Check sheet for the modelled part. Datum: model origin and axes. Units: mm. A direction names the side the tool comes from. Coordinates: 2 decimals unless noted, no trailing zeros. Write each loop counter-clockwise with the first axis right and the second up, starting at its lowest first coordinate (ties: lowest second). Pieces come first, ordered by that corner, then holes. Notation, with made-up numbers: (43.5, 6) -> (67.5, 6) arc R28 ccw to (67.5, 40) -> close; hole circle Ø4 at (63.25, 25). An arc over 180 degrees is marked (long way). One line per item, written item: value. Start each with the question number.
1) Sectioned sample at C-C on y = -4.75. Give the number of separate pieces and of enclosed holes in the cut face, plus the area to 3 significant figures.
2) Gauge pin test, flat ends, axial feed: P1, Ø1.5, axis at x = -12, y = -15, coming from the -Z side; P2, Ø4, axis at x = 34.5, z = -45.5, coming from the -Y side; P3, Ø8, axis at x = 9, y = -6.5, coming from the +Z side. Record the tip position at first contact, or that the pin passes through.
3) Scan lines: line 1 along Z through (x, y) = (0, -0.3); line 2 along X through (y, z) = (-17.75, -22.5); line 3 along Z through (x, y) = (-41, -12). Record each from-to range of solid material in increasing order. Write a range as [from, to].
4) Sectioned sample at D-D on x = -44. Enter the section's corners in (y, z).
5) Sectioned sample at B-B on z = 0. Enter the section's corners in (x, y).
6) Draft check along Z on faces 1 (the cylindrical face through (-35.48, -12.83, 51.01)), 2 (the flat face through (30, -25, 40)), 3 (the flat face through (43.919, -12.832, 3.362)). Enter one of: +Z half, -Z half, draft (parallel to the pull), parting line (faces both ways), or undercut.
7) Sectioned sample at A-A on x = 0. Enter the section's corners in (y, z), plus the area to 3 significant figures.
8) Set-up check for faces 4 (the flat face through (-34.05, -12.83, -27.95)), 5 (the flat face through (10, -13, 43)), 6 (the cylindrical face through (27.912, -13.168, -19.875)), 7 (the flat face through (-23, -25, -30)): record each of +Z, -Z, +X, -X, +Y, -Y from which the full face is reachable in a straight line by a thin tool's end or side.
```python
from build123d import *

# Parameters (mm, degrees)
F0_R     = 68.635064
F0_R_2   = 2.1
F0_R_3   = 28.5
F1_DEPTH = 1
F2_DEPTH = 25
F3_R     = 10


with BuildPart() as f1:
    # F0 (on Front) → F1 (new body)
    with BuildSketch(Plane.XZ):
        Circle(F0_R)
        with Locations((-22.828554, -29.75075)):
            Circle(F0_R_2, mode=Mode.SUBTRACT)
        with Locations((21.509116, -30.718202)):
            Circle(F0_R_2, mode=Mode.SUBTRACT)
        with BuildLine():
            ThreePointArc((-10, 30.923292), (0, 32.5), (10, 30.923292))
            Line((10, 30.923292), (10, 61.325086))
            ThreePointArc((10, 61.325086), (36.741063, 50.108487), (55.479716, 27.977979))
            Line((55.479716, 27.977979), (26.48501, 18.835983))
            ThreePointArc((26.48501, 18.835983), (30.959755, 9.886536), (32.5, 0))
            ThreePointArc((32.5, 0), (32.499781, -0.119179), (32.499126, -0.238356))
            Line((32.499126, -0.238356), (61.493832, 8.90364))
            ThreePointArc((61.493832, 8.90364), (58.837564, -19.972662), (43.366145, -44.498805))
            Line((43.366145, -44.498805), (25.928392, -19.595114))
            ThreePointArc((25.928392, -19.595114), (18.641234, -26.622441), (9.545351, -31.066642))
            Line((9.545351, -31.066642), (26.983104, -55.970334))
            ThreePointArc((26.983104, -55.970334), (-1.355469, -62.120278), (-29.398814, -54.740076))
            Line((-29.398814, -54.740076), (-10.891374, -30.620711))
            ThreePointArc((-10.891374, -30.620711), (-19.784746, -25.783984), (-26.758441, -18.445483))
            Line((-26.758441, -18.445483), (-45.265881, -42.564848))
            ThreePointArc((-45.265881, -42.564848), (-59.652759, -17.387194), (-61.046932, 11.577489))
            Line((-61.046932, 11.577489), (-32.478591, 1.179463))
            ThreePointArc((-32.478591, 1.179463), (-30.54001, 11.115655), (-25.638188, 19.973315))
            Line((-25.638188, 19.973315), (-54.20653, 30.371341))
            ThreePointArc((-54.20653, 30.371341), (-35.639209, 50.898065), (-10, 61.325086))
            Line((-10, 61.325086), (-10, 30.923292))
        make_face(mode=Mode.SUBTRACT)
        with Locations((-35.238473, 12.825755)):
            Circle(F0_R_2, mode=Mode.SUBTRACT)
        with Locations((35.764386, 11.276467)):
            Circle(F0_R_2, mode=Mode.SUBTRACT)
        with Locations((0, 37.5)):
            Circle(F0_R_2, mode=Mode.SUBTRACT)
        with BuildLine():
            Line((10, 61.325086), (10, 30.923292))
            ThreePointArc((10, 30.923292), (19.217564, 26.20945), (26.48501, 18.835983))
            Line((26.48501, 18.835983), (55.479716, 27.977979))
            ThreePointArc((55.479716, 27.977979), (36.741063, 50.108487), (10, 61.325086))
        make_face()
        with BuildLine():
            ThreePointArc((-25.638188, 19.973315), (-18.641234, 26.622441), (-10, 30.923292))
            Line((-10, 30.923292), (-10, 61.325086))
            ThreePointArc((-10, 61.325086), (-35.639209, 50.898065), (-54.20653, 30.371341))
            Line((-54.20653, 30.371341), (-25.638188, 19.973315))
        make_face()
        with Locations((0, 37.5)):
            Circle(F0_R_2)
        with Locations((35.764386, 11.276467)):
            Circle(F0_R_2)
        with BuildLine():
            Line((61.493832, 8.90364), (32.499126, -0.238356))
            ThreePointArc((32.499126, -0.238356), (30.775229, -10.446783), (25.928392, -19.595114))
            Line((25.928392, -19.595114), (43.366145, -44.498805))
            ThreePointArc((43.366145, -44.498805), (58.837564, -19.972662), (61.493832, 8.90364))
        make_face()
        with BuildLine():
            Line((26.983104, -55.970334), (9.545351, -31.066642))
            ThreePointArc((9.545351, -31.066642), (-0.708984, -32.492266), (-10.891374, -30.620711))
            Line((-10.891374, -30.620711), (-29.398814, -54.740076))
            ThreePointArc((-29.398814, -54.740076), (-1.355469, -62.120278), (26.983104, -55.970334))
        make_face()
        with BuildLine():
            ThreePointArc((-26.758441, -18.445483), (-31.20162, -9.094443), (-32.478591, 1.179463))
            Line((-32.478591, 1.179463), (-61.046932, 11.577489))
            ThreePointArc((-61.046932, 11.577489), (-59.652759, -17.387194), (-45.265881, -42.564848))
            Line((-45.265881, -42.564848), (-26.758441, -18.445483))
        make_face()
        with Locations((-35.238473, 12.825755)):
            Circle(F0_R_2)
        with BuildLine():
            ThreePointArc((26.48501, 18.835983), (19.217564, 26.20945), (10, 30.923292))
            ThreePointArc((10, 30.923292), (0, 32.5), (-10, 30.923292))
            ThreePointArc((-10, 30.923292), (-18.641234, 26.622441), (-25.638188, 19.973315))
            ThreePointArc((-25.638188, 19.973315), (-30.54001, 11.115655), (-32.478591, 1.179463))
            ThreePointArc((-32.478591, 1.179463), (-31.20162, -9.094443), (-26.758441, -18.445483))
            ThreePointArc((-26.758441, -18.445483), (-19.784746, -25.783984), (-10.891374, -30.620711))
            ThreePointArc((-10.891374, -30.620711), (-0.708984, -32.492266), (9.545351, -31.066642))
            ThreePointArc((9.545351, -31.066642), (18.641234, -26.622441), (25.928392, -19.595114))
            ThreePointArc((25.928392, -19.595114), (30.775229, -10.446783), (32.499126, -0.238356))
            ThreePointArc((32.499126, -0.238356), (32.499781, -0.119179), (32.5, 0))
            ThreePointArc((32.5, 0), (30.959755, 9.886536), (26.48501, 18.835983))
        make_face()
        Circle(F0_R_3, mode=Mode.SUBTRACT)
        with Locations((21.509116, -30.718202)):
            Circle(F0_R_2)
        with Locations((-22.828554, -29.75075)):
            Circle(F0_R_2)
    extrude(amount=F1_DEPTH)

    # F0 (on Front) → F2 (join)
    with BuildSketch(Plane.XZ):
        with BuildLine():
            Line((10, 61.325086), (10, 30.923292))
            ThreePointArc((10, 30.923292), (19.217564, 26.20945), (26.48501, 18.835983))
            Line((26.48501, 18.835983), (55.479716, 27.977979))
            ThreePointArc((55.479716, 27.977979), (36.741063, 50.108487), (10, 61.325086))
        make_face()
        with BuildLine():
            ThreePointArc((-25.638188, 19.973315), (-18.641234, 26.622441), (-10, 30.923292))
            Line((-10, 30.923292), (-10, 61.325086))
            ThreePointArc((-10, 61.325086), (-35.639209, 50.898065), (-54.20653, 30.371341))
            Line((-54.20653, 30.371341), (-25.638188, 19.973315))
        make_face()
        with BuildLine():
            ThreePointArc((-26.758441, -18.445483), (-31.20162, -9.094443), (-32.478591, 1.179463))
            Line((-32.478591, 1.179463), (-61.046932, 11.577489))
            ThreePointArc((-61.046932, 11.577489), (-59.652759, -17.387194), (-45.265881, -42.564848))
            Line((-45.265881, -42.564848), (-26.758441, -18.445483))
        make_face()
        with BuildLine():
            Line((26.983104, -55.970334), (9.545351, -31.066642))
            ThreePointArc((9.545351, -31.066642), (-0.708984, -32.492266), (-10.891374, -30.620711))
            Line((-10.891374, -30.620711), (-29.398814, -54.740076))
            ThreePointArc((-29.398814, -54.740076), (-1.355469, -62.120278), (26.983104, -55.970334))
        make_face()
        with BuildLine():
            Line((61.493832, 8.90364), (32.499126, -0.238356))
            ThreePointArc((32.499126, -0.238356), (30.775229, -10.446783), (25.928392, -19.595114))
            Line((25.928392, -19.595114), (43.366145, -44.498805))
            ThreePointArc((43.366145, -44.498805), (58.837564, -19.972662), (61.493832, 8.90364))
        make_face()
        with Locations((35.764386, 11.276467)):
            Circle(F0_R_2)
        with Locations((21.509116, -30.718202)):
            Circle(F0_R_2)
        with Locations((-22.828554, -29.75075)):
            Circle(F0_R_2)
        with Locations((-35.238473, 12.825755)):
            Circle(F0_R_2)
        with Locations((0, 37.5)):
            Circle(F0_R_2)
    extrude(amount=F2_DEPTH)

    # F3
    f3_edges = [f1.edges().sort_by_distance(p)[0] for p in [
        (-54.20653, -13, 30.371341),
        (-25.638188, -13, 19.973315),
        (-10, -13, 30.923292),
        (-10, -13, 61.325086),
        (-32.478591, -13, 1.179463),
        (-26.758441, -13, -18.445483),
        (-61.046932, -13, 11.577489),
        (-45.265881, -13, -42.564848),
        (-29.398814, -13, -54.740076),
        (26.983104, -13, -55.970334),
        (9.545351, -13, -31.066642),
        (-10.891374, -13, -30.620711),
        (32.499126, -13, -0.238356),
        (25.928392, -13, -19.595114),
        (43.366145, -13, -44.498805),
        (61.493832, -13, 8.90364),
        (55.479716, -13, 27.977979),
        (10, -13, 61.325086),
        (10, -13, 30.923292),
        (26.48501, -13, 18.835983),
    ]]
    fillet(f3_edges, radius=F3_R)


solid = f1.part
```
Answers:
1. separate pieces: 10
1. enclosed holes: 0
1. area: 5,390 mm2
2. P1: stops at z = -61.11
2. P2: stops at y = -1
2. P3: stops at z = 55.29
3. line 1: z = [-68.64, -28.5], [28.5, 68.64]
3. line 2: x = [-57.92, -29.99], [28.44, 57.92]
3. line 3: z = [-35.11, 4.28], [25.56, 46.69]
4. outline: (-25, -35.95) -> (-1, -35.95) -> (-1, -52.68) -> (0, -52.68) -> (0, 52.68) -> (-1, 52.68) -> (-1, 43.87) -> (-25, 43.87) -> (-25, 26.97) -> (-1, 26.97) -> (-1, 5.37) -> (-25, 5.37) -> close
5. outline: (-68.64, -1) -> (-61.81, -1) -> (-61.81, -25) -> (-34.06, -25) -> (-34.06, -1) -> (-28.5, -1) -> (-28.5, 0) -> (-68.64, 0) -> close; (28.5, -1) -> (35.52, -1) -> (35.52, -25) -> (60.81, -25) -> (60.81, -1) -> (68.64, -1) -> (68.64, 0) -> (28.5, 0) -> close
6. face 1: +Z half
6. face 2: draft
6. face 3: undercut
7. outline: (-25, -62.14) -> (-1, -62.14) -> (-1, -68.64) -> (0, -68.64) -> (0, -28.5) -> (-1, -28.5) -> (-1, -32.5) -> (-25, -32.5) -> close; (-25, 35.4) -> (-1, 35.4) -> (-1, 28.5) -> (0, 28.5) -> (0, 68.64) -> (-1, 68.64) -> (-1, 39.6) -> (-25, 39.6) -> close
7. area: 892 mm2
8. face 4: -Z, -Y
8. face 5: +Z, -Y
8. face 6: -Y
8. face 7: +Z, -Z, +X, -X, -Y
